Autodesk Inventor part; units mm, degrees
ref_plane "Work Plane1" through (0, 0, -15) normal (0, 0, 1) x (1, 0, 0)
ref_plane "YZ Plane" through (0, 0, 0) normal (1, 0, 0) x (0, 1, 0)
ref_plane "XZ Plane" through (0, 0, 0) normal (0, 1, 0) x (-1, 0, 0)
sketch "Sketch1" plane through (0, 0, 0) normal (0, 0, 1) x (1, 0, 0)
  line L0 (0, 0) -> (25, 0)
  line L1 (25, 0) -> (25, 40)
  line L2 (25, 40) -> (0, 40)
  line L3 (0, 40) -> (0, 0)
  dimension "d1" = 25
  dimension "d2" = 40
  dimension "d3" = 25
extrude "Extrusion1" add sketch "Sketch1" against normal blind 30
sketch "Sketch2" plane through (25, 0, 0) normal (1, 0, 0) x (0, 0, -1)
  line L0 (0, 0) -> (30, 0)
  circle A0 centre (15, 6.56) radius 2.46
extrude "Extrusion2" cut sketch "Sketch2" against normal blind 30
sketch "Sketch3" plane through (0, 0, 0) normal (-1, 0, 0) x (0, 0, 1)
  line L0 (0, 0) -> (-30, 0)
  line L1 (-25.05, 0) -> (-4.95, 0)
  line L2 (-4.95, 0) -> (-4.95, 33.12)
  line L3 (-4.95, 33.12) -> (-25.05, 33.12)
  line L4 (-25.05, 33.12) -> (-25.05, 0)
  dimension "d11" = 20.1
extrude "Extrusion3" cut sketch "Sketch3" against normal blind 20
sketch "Sketch4" plane through (0, 0, 0) normal (0, -1, 0) x (1, 0, 0)
  line L0 (20, -4.95) -> (20, -25.05)
  line L1 (20, -15) -> (25, -15)
  line L2 (25, 0) -> (25, -30)
  line L3 (20, -8.025) -> (25, -8.025)
  line L4 (25, -8.025) -> (25, -21.975)
  line L5 (25, -21.975) -> (20, -21.975)
  line L6 (20, -21.975) -> (20, -8.025)
  line L7 (20, -8.025) -> (25, -21.975) construction
  line L8 (25, -8.025) -> (20, -21.975) construction
  line L9 (25, -12.54) -> (25, -17.46)
  point P0 (0, 0)
  point P1 (22.5, -15)
  dimension "d14" = 13.95
extrude "Extrusion4" add sketch "Sketch4" along normal blind 15
sketch "Sketch5" plane through (20, 0, 0) normal (-1, 0, 0) x (0, 0, 1)
  circle A0 centre (-15, 6.56) radius 2.46
  circle A1 centre (-15, 6.56) radius 4.7025
  circle A2 centre (-15, 6.56) radius 2.46
  circle A3 centre (-15, 6.56) radius 2.46
  point P0 (0, 0)
  dimension "d17" = 9.405
extrude "Extrusion5" cut sketch "Sketch5" against normal blind 2.1
sketch "Sketch6" plane through (25, 0, 0) normal (1, 0, 0) x (0, 0, -1)
  circle A0 centre (15, 6.56) radius 4.7025
  line L0 (15, 6.56) -> (15, 23.56)
  circle A1 centre (15, 23.56) radius 2.46
  point P0 (0, 0)
  dimension "d20" = 17
  dimension "d21" = 4.92
extrude "Extrusion6" cut sketch "Sketch6" against normal blind 10 contours A1
sketch "Sketch7" plane through (20, 0, 0) normal (-1, 0, 0) x (0, 0, 1)
  circle A0 centre (-15, 23.56) radius 2.46
  circle A1 centre (-15, 23.56) radius 4.7025
  point P0 (0, 0)
  dimension "d24" = 9.405
extrude "Extrusion7" cut sketch "Sketch7" against normal blind 2.1
sketch "Sketch9" plane through (25, 0, 0) normal (1, 0, 0) x (0, 0, -1)
  circle A0 centre (15, 6.56) radius 2.46
  circle A1 centre (15, 6.56) radius 2.46
  circle A2 centre (15, 23.56) radius 2.46
  circle A3 centre (15, 23.56) radius 2.46
  line L0 (30, 40) -> (30, 0)
  line L1 (30, 0) -> (30, 40)
  line L2 (30, 40) -> (0, 40)
  line L3 (0, 40) -> (0, 0)
  line L4 (0, 0) -> (8.025, 0)
  line L5 (21.975, 0) -> (21.975, -15)
  line L6 (21.975, -15) -> (8.025, -15)
  line L7 (8.025, -15) -> (8.025, 0)
  line L8 (0, 0) -> (8.025, 0)
  line L9 (21.975, 0) -> (30, 0)
extrude "Extrusion8" add sketch "Sketch9" along normal blind 5
sketch "Sketch10" plane through (0, 40, 0) normal (0, 1, 0) x (1, 0, 0)
  line L0 (0, 30) -> (30, 30)
  line L1 (30, 0) -> (0, 0)
  line L2 (0, 30) -> (30, 30)
  line L3 (30, 30) -> (30, 0)
  line L4 (30, 0) -> (0, 0)
  line L5 (0, 0) -> (0, 30)
extrude "Extrusion9" add sketch "Sketch10" along normal blind 30
sketch "Sketch12" plane through (30, 0, 0) normal (1, 0, 0) x (0, 0, -1)
  circle A0 centre (15, 6.56) radius 2.46
  line L0 (15, 6.56) -> (15, 15.06)
  circle A1 centre (15, 15.06) radius 2.525
  point P0 (0, 0)
  dimension "d31" = 8.5
  dimension "d33" = 5.05
extrude "Extrusion10" cut sketch "Sketch12" against normal blind 30 contours A1
sketch "Sketch15" plane through (0, 0, -25.05) normal (-1, 0, 0) x (0, 0, 1)
  line L0 (0, 33.12) -> (20.1, 33.12)
  line L1 (20.1, 33.12) -> (20.1, 0)
  line L2 (0, 33.12) -> (20.1, 33.12)
  line L3 (20.1, 33.12) -> (20.1, 31.1)
  line L4 (20.1, 31.1) -> (0, 31.1)
  line L5 (0, 31.1) -> (0, 33.12)
  point P0 (25.05, 0)
  dimension "d57" = 2.02
extrude "Extrusion13" add sketch "Sketch15" against normal blind 20
sketch "Sketch17" plane through (0, 0, 0) normal (0, 0, 1) x (1, 0, 0)
  line L0 (0, 70) -> (30, 70)
  line L1 (30, 70) -> (50.0622, 90.0622)
  line L2 (30, 70) -> (80, 70) construction
  line L3 (11.9522, 97.2454) -> (0, 85.2932)
  line L4 (0, 70) -> (0, 85.2932)
  line L5 (0, 70) -> (0, 0)
  line L6 (0, 70) -> (30, 70)
  line L7 (10.923, 112.2849) -> (0, 120.567)
  line L8 (50.0622, 105.3553) -> (50.0622, 120.567)
  line L9 (50.0622, 105.3553) -> (50.0622, 90.0622)
  arc A0 (11.9522, 97.2454) -> (10.923, 112.2849) centre (4.8811, 104.3165) ccw
  line L10 (0, 152.567) -> (30, 152.567)
  line L11 (30, 152.567) -> (50.0622, 120.567)
  line L12 (5, 150.567) -> (0, 152.567)
  line L13 (5, 122.567) -> (0, 120.567)
  line L14 (5, 122.567) -> (10, 136.567)
  line L15 (10, 136.567) -> (5, 150.567)
  dimension "d61" = 45
  dimension "d62" = 32.0271
  dimension "d72" = 10
extrude "Extrusion14" add sketch "Sketch17" against normal blind 30
sketch "Sketch22" plane through (0, 0, 0) normal (0, 0, 1) x (1, 0, 0)
  line L0 (30, 0) -> (30, 70)
  line L1 (50.0622, 90.0622) -> (30, 70)
  line L2 (30, 70) -> (50.0622, 90.0622)
  line L3 (50.0622, 120.567) -> (50.0622, 90.0622)
  line L4 (50.0622, 90.0622) -> (50.0622, 120.567)
  line L5 (30, 152.567) -> (50.0622, 120.567)
  line L6 (50.0622, 120.567) -> (30, 152.567)
  line L7 (0, 152.567) -> (30, 152.567)
  line L8 (30, 152.567) -> (0, 152.567)
  line L9 (5, 150.567) -> (0, 152.567)
  line L10 (0, 152.567) -> (5, 150.567)
  line L11 (5, 150.567) -> (10, 136.567)
  line L12 (5, 150.567) -> (10, 136.567)
  line L13 (10, 136.567) -> (5, 122.567)
  line L14 (10, 136.567) -> (5, 122.567)
  line L15 (5, 122.567) -> (0, 120.567)
  line L16 (5, 122.567) -> (0, 120.567)
  line L17 (0, 120.567) -> (10.923, 112.2849)
  line L18 (0, 120.567) -> (10.923, 112.2849)
  line L19 (0, 85.2932) -> (11.9522, 97.2454)
  line L20 (11.9522, 97.2454) -> (0, 85.2932)
  line L21 (0, 85.2932) -> (0, 55.2932)
  line L22 (0, 0) -> (0, 85.2932)
  line L23 (0, 55.2932) -> (30, 55.2932)
  line L24 (30, 55.2932) -> (30, 70)
  arc A0 (11.9522, 97.2454) -> (10.923, 112.2849) centre (4.8811, 104.3165) ccw
  dimension "d92" = 30
extrude "Extrusion15" add sketch "Sketch22" along normal blind 15
ref_plane "Work Plane1" through (0, 0, -15) normal (0, 0, 1) x (1, 0, 0)
mirror "Mirror1" about plane through (0, 0, -15) normal (0, 0, 1) of "Extrusion15"
properties part number "rec_c_28mm_x_60mm"
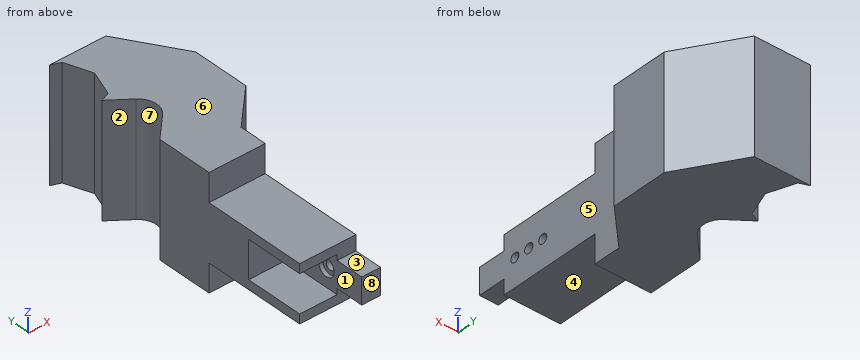
CAD build for the part. Positions are in the model's coordinates, mm. Face numbers are marked on the shaded views. A direction names the side the tool comes from. Round coordinates to 2 decimals unless told otherwise and drop trailing zeros. Order: outer loops, then holes, each group sorted by start corner. A loop starts at its lowest first (then second) coordinate and runs counter-clockwise, first axis right, second up.
Item 1: Saw through at B-B on z = 6. Write the cut outline in (x, y), then the cut area to 3 significant figures.
Item 2: Pin check, flat tips, straight feed: pin 1 (1 mm diameter, centred on y = 19, z = -3, fed in from +X); pin 2 (2 mm diameter, centred on x = 43.5, z = -25, fed in from -Y); pin 3 (5 mm diameter, centred on x = 5, y = 24.5, fed in from +Z); pin 4 (10 mm diameter, centred on x = 5.5, y = 113.5, fed in from -Z). Stop position of each tip, or through.
Item 3: Tool access for the marked faces 1, 2, 3, 4 and 5: list every direction of +Z, -Z, +X, -X, +Y, -Y with a clear straight run to the whole face (end or side of a thin tool).
Item 4: Saw through at D-D on z = -15. State how many separate pieces and enclosed holes the cut face has, then the cut area to 3 significant figures.
Item 5: Probe line 1 along Z through (x, y) = (26.25, 23.56); line 2 along Y through (x, z) = (25, -15) (3 decimals); line 3 along Y through (x, z) = (20, -41). List the from-to ranges inside material, lowest first.
Item 6: Mould opens along Y. For the marked faces 6, 7 and 8 say: pulls with the +Y half, pulls with the -Y half, needs draft (parallel to the pull), parting line crosses it, or undercut.
Item 7: Saw through at C-C on x = 8. Write the cut outline in (y, z), then the cut area to 3 significant figures.
Item 8: Saw through at A-A on y = 15.06. Write the cut outline in (x, z) (3 decimals).
Reported:
1. outline: (0, 55.29) - (30, 55.29) - (30, 70) - (50.06, 90.06) - (50.06, 120.57) - (30, 152.57) - (0, 152.57) - (5, 150.57) - (10, 136.57) - (5, 122.57) - (0, 120.57) - (10.92, 112.28) arc R10 cw to (11.95, 97.25) - (0, 85.29) - close
1. area: 3,510 mm2
2. pin 1: stops at x = 30
2. pin 2: stops at y = 82.5
2. pin 3: stops at z = 0
2. pin 4: stops at z = -45
3. face 1: -X, -Y
3. face 2: +Z, -Z, -X
3. face 3: +Z, +X, -X, -Y
3. face 4: -Z, +X, -X, -Y
3. face 5: +Z, -Z, +X, -Y
4. separate pieces: 4
4. enclosed holes: 0
4. area: 4,530 mm2
5. line 1: z = -30 to -17.46, -12.54 to 0
5. line 2: y = -15 to 4.1, 9.02 to 12.535, 17.585 to 21.1, 26.02 to 152.567
5. line 3: y = 55.29 to 152.57
6. face 6: needs draft
6. face 7: undercut
6. face 8: pulls with the -Y half
7. outline: (0, -30) - (55.29, -30) - (55.29, -45) - (93.29, -45) - (93.29, 15) - (55.29, 15) - (55.29, 0) - (0, 0) - (0, -4.95) - (31.1, -4.95) - (31.1, -25.05) - (0, -25.05) - close; (114.5, -45) - (130.97, -45) - (130.97, 15) - (114.5, 15) - close; (142.17, -45) - (152.57, -45) - (152.57, 15) - (142.17, 15) - close
7. area: 4,930 mm2
8. outline: (0, -30) - (30, -30) - (30, -17.525) - (20, -17.525) - (20, -25.05) - (0, -25.05) - close; (0, -4.95) - (20, -4.95) - (20, -12.475) - (30, -12.475) - (30, 0) - (0, 0) - close
